Source: CAD feature listing. Evaluate the final solid. Frame: model axes, mm. Give positions to 0.01 mm unless a question says otherwise; leave off trailing zeros. Loops run counter-clockwise (first coordinate to the right, second up) from the corner with the lowest first, then second, coordinate; pieces in that order, holes last. Notation, with made-up numbers: (76.5, 10) -> (112.5, 10) arc R11 cw to (112.5, 15) -> close; hole circle Ø3 at (19.5, 59). An arc over 180 degrees is marked (long way). Put each result on its own line as item: value.
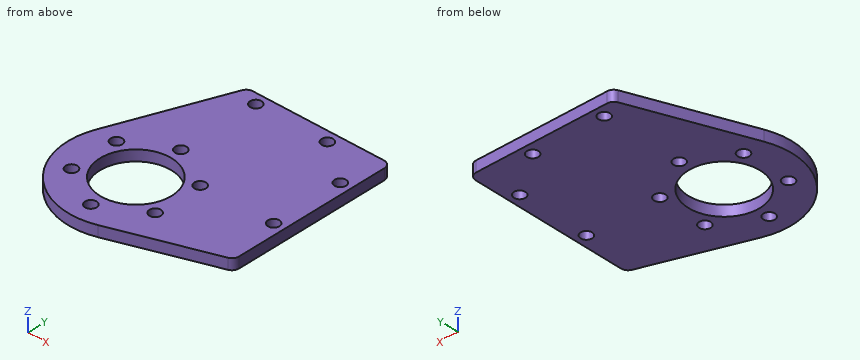
```python
from build123d import *

# Parameters (mm, degrees)
SKETCH_1_R      = 19
SKETCH_1_R_2    = 10
SKETCH_1_R_3    = 1.6
EXTRUDE_1_DEPTH = 3
EXTRUDE_START   = -3
SKETCH_2_R      = 1.6
EXTRUDE_3_DEPTH = 3


with BuildPart() as part:
    # 草图1 → 凸台-拉伸1 (new body)
    with BuildSketch(Plane.XY):
        Circle(SKETCH_1_R)
        Circle(SKETCH_1_R_2, mode=Mode.SUBTRACT)
        with Locations((0, 13.5)):
            Circle(SKETCH_1_R_3, mode=Mode.SUBTRACT)
        with Locations((11.691342951, 6.75)):
            Circle(SKETCH_1_R_3, mode=Mode.SUBTRACT)
        with Locations((11.691342951, -6.75)):
            Circle(SKETCH_1_R_3, mode=Mode.SUBTRACT)
        with Locations((0, -13.5)):
            Circle(SKETCH_1_R_3, mode=Mode.SUBTRACT)
        with Locations((-11.691342951, -6.75)):
            Circle(SKETCH_1_R_3, mode=Mode.SUBTRACT)
        with Locations((-11.691342951, 6.75)):
            Circle(SKETCH_1_R_3, mode=Mode.SUBTRACT)
    extrude(amount=EXTRUDE_1_DEPTH)

    # 草图2 → 凸台-拉伸3 (add)
    with BuildSketch(Plane.XY.offset(3).offset(EXTRUDE_START)):
        with BuildLine():
            Line((35, -6.575441021), (35, 37))
            ThreePointArc((35, 37), (34.414213562, 38.414213562), (33, 39))
            Line((33, 39), (-3.640557622, 39))
            ThreePointArc((-3.640557622, 39), (-4.764862291, 38.654067414), (-5.500233339, 37.735939011))
            Line((-5.500233339, 37.735939011), (-17.666919312, 6.991420601))
            ThreePointArc((-17.666919312, 6.991420601), (13.726454821, 13.137139645), (6.209937899, -17.956521692))
            Line((6.209937899, -17.956521692), (33.653677674, -8.4656012))
            ThreePointArc((33.653677674, -8.4656012), (34.629011256, -7.735752327), (35, -6.575441021))
        make_face()
        with Locations((32, 7)):
            Circle(SKETCH_2_R, mode=Mode.SUBTRACT)
        with Locations((32, 27)):
            Circle(SKETCH_2_R, mode=Mode.SUBTRACT)
        with Locations((0, 36)):
            Circle(SKETCH_2_R, mode=Mode.SUBTRACT)
        with Locations((20, 36)):
            Circle(SKETCH_2_R, mode=Mode.SUBTRACT)
    extrude(amount=EXTRUDE_3_DEPTH)


solid = part.part
```
(1) Section C-C on z = 1.9. Give the number of separate pieces and of enclosed holes in the cut face, then the cut area to 3 significant figures.
Calculated:
separate pieces: 1
enclosed holes: 11
area: 2,230 mm²
(2) Line query: probe 1 along Y at (x, z) = (0, 0.8); probe 2 along Y at (x, z) = (32, 1.3); probe 3 along Y at (x, z) = (1, 0.5). Output: solid intervals per line, ascending. Write a range as from..to.
Calculated:
probe 1: y = -19..-15.1, -11.9..-10, 10..11.9, 15.1..34.4, 37.6..39
probe 2: y = -9.04..5.4, 8.6..25.4, 28.6..39
probe 3: y = -18.97..-14.75, -12.25..-9.95, 9.95..12.25, 14.75..34.75, 37.25..39
(3) First-contact query: P1, Ø1, axis at y = 1, z = 1.5, coming from the -X side; P2, Ø3, axis at x = 32, y = 27, coming from the +Z side. Flat tips, straight axial feed; report the tip coordinate or a pass-through.
Calculated:
P1: stops at x = -18.99
P2: passes through
(4) Section A-A on y = 0. Return loops of the section in (x, z).
Calculated:
outline: (-19, 0) -> (-10, 0) -> (-10, 3) -> (-19, 3) -> close; (10, 0) -> (35, 0) -> (35, 3) -> (10, 3) -> close
(5) Section B-B on x = 0. Return loops of the section in (y, z).
Calculated:
outline: (-19, 0) -> (-15.1, 0) -> (-15.1, 3) -> (-19, 3) -> close; (-11.9, 0) -> (-10, 0) -> (-10, 3) -> (-11.9, 3) -> close; (10, 0) -> (11.9, 0) -> (11.9, 3) -> (10, 3) -> close; (15.1, 0) -> (34.4, 0) -> (34.4, 3) -> (15.1, 3) -> close; (37.6, 0) -> (39, 0) -> (39, 3) -> (37.6, 3) -> close
(6) Section D-D on x = 32. Return loops of the section in (y, z).
Calculated:
outline: (-9.04, 0) -> (5.4, 0) -> (5.4, 3) -> (-9.04, 3) -> close; (8.6, 0) -> (25.4, 0) -> (25.4, 3) -> (8.6, 3) -> close; (28.6, 0) -> (39, 0) -> (39, 3) -> (28.6, 3) -> close
